```python
from build123d import *

# Parameters (mm, degrees)
PAD_DEPTH    = 140
SKETCH001_W  = 120
SKETCH001_H  = 140
PAD001_DEPTH = 40
POCKET_DEPTH = 157.501


with BuildPart() as part:
    # Sketch → Pad (new body)
    with BuildSketch(Plane.XZ):
        Polygon((0, 0), (37.5, 22), (157.5, 22), (195, 0), (195, -35), (160, -35), (160, 0), (142.954545, 10), (52.045455, 10), (35, 0), (35, -35), (0, -35), align=None)
        with BuildLine():
            Line((7.400011, -9.4), (7.400011, -25.6))
            ThreePointArc((7.400011, -25.6), (7.985793, -27.01421), (9.4, -27.6))
            Line((9.4, -27.6), (25.6, -27.6))
            ThreePointArc((25.6, -27.6), (27.014214, -27.014214), (27.6, -25.6))
            Line((27.6, -9.4), (27.6, -25.6))
            ThreePointArc((27.6, -9.4), (27.014214, -7.985786), (25.6, -7.4))
            Line((9.4, -7.4), (25.6, -7.4))
            ThreePointArc((9.4, -7.4), (7.985793, -7.98579), (7.400011, -9.4))
        make_face(mode=Mode.SUBTRACT)
        with BuildLine():
            Line((169.4, -7.4), (185.6, -7.4))
            ThreePointArc((187.6, -9.4), (187.014214, -7.985786), (185.6, -7.4))
            Line((187.6, -9.4), (187.6, -25.6))
            ThreePointArc((185.6, -27.6), (187.014214, -27.014214), (187.6, -25.6))
            Line((185.6, -27.6), (169.4, -27.6))
            ThreePointArc((167.4, -25.6), (167.985786, -27.014214), (169.4, -27.6))
            Line((167.4, -25.6), (167.4, -9.4))
            ThreePointArc((169.4, -7.4), (167.985786, -7.985786), (167.4, -9.4))
        make_face(mode=Mode.SUBTRACT)
    extrude(amount=PAD_DEPTH)

    # Sketch001 (on Face2 of Pad) → Pad001 (join)
    with BuildSketch(Plane(origin=(0, 0, 22), x_dir=(-1, 0, 0), z_dir=(0, 0, 1))):
        with Locations((-97.5, 70)):
            Rectangle(SKETCH001_W, SKETCH001_H)
    extrude(amount=PAD001_DEPTH)

    # Sketch002 (on Face3 of Pad001) → Pocket (cut, through all)
    with BuildSketch(Plane(origin=(37.5, 0, 0), x_dir=(0, 0, -1), z_dir=(-1, 0, 0))):
        Polygon((-62, 30.100903), (-22, 140), (-62, 140), align=None)
        Polygon((-22, 0), (-62, 0), (-62, 18.531311), align=None)
    extrude(amount=-POCKET_DEPTH, mode=Mode.SUBTRACT)


solid = part.part
```
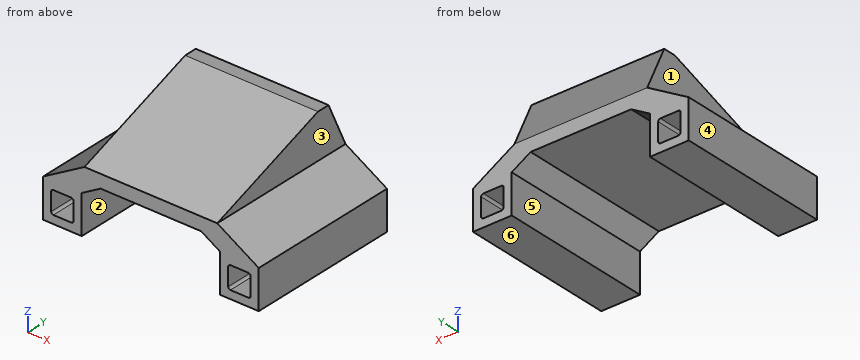
Geometry check sheet. Reference: the model listing, model coordinates, mm. Face numbers are marked on the shaded views. A direction names the side the tool comes from. Round coordinates to 2 decimals unless told otherwise and drop trailing zeros. Order: outer loops, then holes, each group sorted by start corner. A loop starts at its lowest first (then second) coordinate and runs counter-clockwise, first axis right, second up. Notation, with made-up numbers: (-19.75, 15.25) - (26.25, 15.25) arc R15 ccw to (26.25, 36.25) - close; hole circle Ø9 at (87, 29). An arc over 180 degrees is marked (long way). Use a Markdown table: item, result. Add a question column.
(1) Tool access check on the marked faces 1, 2 and 3. Record the directions out of +Z, -Z, +X, -X, +Y, -Y that give a thin tool (end or side, any length) a straight path to the whole face; none if there is none.
(2) Depth check by flat-ended pin: pin 1 (5 mm diameter, centred on x = 17.5, y = -70.5, fed in from +Z); pin 2 (8 mm diameter, centred on x = 83, z = 48, fed in from +Y); pin 3 (3 mm diameter, centred on x = 105.5, y = -80.5, fed in from +Z); pin 4 (18 mm diameter, centred on y = -43, z = -21, fed in from -X). Enter the tip coordinate at first touch or a pass-through.
(3) Sectioned sample at D-D, the plane z = 7. Enter the section's corners in (x, y).
(4) Material ranges on line 1 along X through (y, z) = (-70.5, 32); line 2 along Z through (x, y) = (110, -28); line 3 along X through (y, z) = (-92, -8), recorded low to high. Write a range as [from, to].
(5) Sectioned sample at B-B, the plane y = -129. Count the separate pieces of the cut face and the enclosed holes in it, and give its area (3 significant figures).
(6) Release check for a two-part mould opening along X. For the marked faces 4, 5 and 6 record: pulls with the +X half, pulls with the -X half, needs draft (parallel to the pull), parting line crosses it, or undercut.
(7) Sectioned sample at C-C, the plane x = 125.5. Enter the section's corners in (y, z).
(8) Sectioned sample at A-A, the plane z = -11.5. Enter the section's corners in (x, y), and give its area (3 significant figures).
Answers below:
| question | item | result |
|---|---|---|
| 1 | face 1 | +Z, -X, +Y, -Y |
| 1 | face 2 | -Z, +Y, -Y |
| 1 | face 3 | +Z, +X, +Y, -Y |
| 2 | pin 1 | z = 11.73 |
| 2 | pin 2 | y = -10.19 |
| 2 | pin 3 | z = 44.2 |
| 2 | pin 4 | x = 0 |
| 3 | outline | (11.93, -140) - (46.93, -140) - (46.93, 0) - (11.93, 0) - close; (148.07, -140) - (183.07, -140) - (183.07, 0) - (148.07, 0) - close |
| 4 | line 1 | [37.5, 157.5] |
| 4 | line 2 | [10, 62] |
| 4 | line 3 | [0, 7.97], [27.03, 35], [160, 167.97], [187.03, 195] |
| 5 | separate pieces | 1 |
| 5 | enclosed holes | 2 |
| 5 | area | 4,510 mm² |
| 6 | face 4 | pulls with the -X half |
| 6 | face 5 | undercut |
| 6 | face 6 | needs draft |
| 7 | outline | (-140, 10) - (0, 10) - (0, 22) - (-18.53, 62) - (-30.1, 62) - (-140, 22) - close |
| 8 | outline | (0, -140) - (7.4, -140) - (7.4, 0) - (0, 0) - close; (27.6, -140) - (35, -140) - (35, 0) - (27.6, 0) - close; (160, -140) - (167.4, -140) - (167.4, 0) - (160, 0) - close; (187.6, -140) - (195, -140) - (195, 0) - (187.6, 0) - close |
| 8 | area | 4,140 mm² |
